Verification items for the finished model (mm, model axes). Coordinates: 2 decimals unless noted, no trailing zeros. Order: outer loops, then holes, each group sorted by start corner. A loop starts at its lowest first (then second) coordinate and runs counter-clockwise, first axis right, second up. Notation, with made-up numbers: (24, 67) - (68, 67) arc R14 ccw to (68, 78) - close; hole circle Ø6 at (14.25, -1.75). An arc over 180 degrees is marked (long way). One line per question, with ' | ' between items. Start each with the question number.
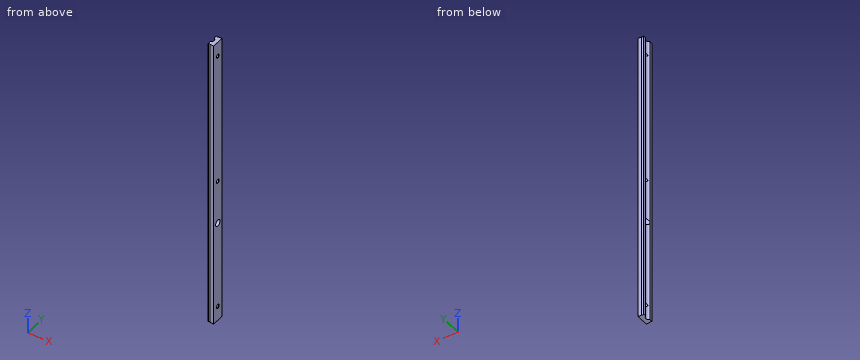
from build123d import *

# Parameters (mm, degrees)
BOSS_EXTRUDE1_DEPTH = 300
SKETCH5_R           = 3.25
CUT_EXTRUDE1_DEPTH  = 6


with BuildPart() as part:
    # Sketch1 → Boss-Extrude1 (new body)
    with BuildSketch(Plane.XY):
        with BuildLine():
            Line((0, 2.974695137), (0, 0))
            Line((0, 0), (0.305572809, 0))
            ThreePointArc((0.305572809, 0), (1.2, 0.4), (2.094427191, 0))
            Line((2.094427191, 0), (5.8, 0))
            Line((5.8, 0), (5.8, 12.1))
            Line((5.8, 12.1), (2.094427191, 12.1))
            ThreePointArc((2.094427191, 12.1), (1.2, 11.7), (0.305572809, 12.1))
            Line((0.305572809, 12.1), (0, 12.1))
            Line((0, 12.1), (0, 9.125304863))
            ThreePointArc((0, 9.125304863), (1.95, 6.05), (0, 2.974695137))
        make_face()
    extrude(amount=BOSS_EXTRUDE1_DEPTH)

    # Sketch2 → Cut-Revolve1 (revolve, cut)
    with BuildSketch(Plane.XY.offset(15), mode=Mode.PRIVATE) as cut_revolve1_sk:
        Polygon((1.299545417, 6.05), (1.299545417, 8.05), (1.678545417, 7.671), (5.421, 7.671), (5.8, 8.05), (5.8, 6.05), align=None)
    revolve(cut_revolve1_sk.sketch.rotate(Axis((5.8, 6.05, 15), (-1, 0, 0)), 270), axis=Axis((5.8, 6.05, 15), (-1, 0, 0)), mode=Mode.SUBTRACT)

    # Sketch3 → Cut-Revolve2 (revolve, cut)
    with BuildSketch(Plane.XY.offset(285), mode=Mode.PRIVATE) as cut_revolve2_sk:
        Polygon((1.299545417, 6.05), (1.299545417, 8.05), (1.678545417, 7.671), (5.421, 7.671), (5.8, 8.05), (5.8, 6.05), align=None)
    revolve(cut_revolve2_sk.sketch.rotate(Axis((5.8, 6.05, 285), (-1, 0, 0)), 270), axis=Axis((5.8, 6.05, 285), (-1, 0, 0)), mode=Mode.SUBTRACT)

    # Sketch4 → Cut-Revolve3 (revolve, cut)
    with BuildSketch(Plane.XY.offset(150), mode=Mode.PRIVATE) as cut_revolve3_sk:
        Polygon((1.299545417, 6.05), (1.299545417, 8.05), (1.678545417, 7.671), (5.421, 7.671), (5.8, 8.05), (5.8, 6.05), align=None)
    revolve(cut_revolve3_sk.sketch.rotate(Axis((5.8, 6.05, 150), (-1, 0, 0)), 270), axis=Axis((5.8, 6.05, 150), (-1, 0, 0)), mode=Mode.SUBTRACT)

    # Sketch5 → Cut-Extrude1 (cut)
    with BuildSketch(Plane(origin=(5.8, 0, 0), x_dir=(0, 0, -1), z_dir=(1, 0, 0))):
        with Locations((-105, 6.05)):
            Circle(SKETCH5_R)
    extrude(amount=-CUT_EXTRUDE1_DEPTH, mode=Mode.SUBTRACT)


solid = part.part
Item 1: Gauge pin test, flat ends, axial feed: pin 1 (3.5 mm diameter, centred on y = 6.05, z = 150, fed in from +X); pin 2 (1 mm diameter, centred on x = 1, z = 256.5, fed in from -Y). Record the tip position at first contact, or that the pin passes through.
Item 2: Thickness scan on probe 1 along Z at (x, y) = (4.3, 6.25); probe 2 along Y at (x, z) = (2.65, 105); probe 3 along Z at (x, y) = (2.6, 6.75). Record the ranges inside material, lowest first. Write a range as from..to.
Item 3: Section check A-A (z = 54.5). Record the cut outline in (x, y).
Completed:
1) pin 1: stops at x = 5.55 | pin 2: stops at y = 0.17
2) probe 1: z = 0..13.39, 16.61..101.76, 108.24..148.39, 151.61..283.39, 286.61..300 | probe 2: y = 0..2.8, 9.3..12.1 | probe 3: z = 0..13.54, 16.46..101.83, 108.17..148.54, 151.46..283.54, 286.46..300
3) outline: (0, 0) - (0.31, 0) arc R1.2 cw to (2.09, 0) - (5.8, 0) - (5.8, 12.1) - (2.09, 12.1) arc R1.2 cw to (0.31, 12.1) - (0, 12.1) - (0, 9.13) arc R3.4 cw to (0, 2.97) - close
